```python
from build123d import *

# Parameters (mm, degrees)
F0_W     = 111
F0_H     = 7
F2_W     = 4.5
F2_H     = 2.05
F3_DEPTH = 12.5
F4_SIZE  = 0.5


with BuildPart() as f1:
    # F0 (on Front) → F1 (revolve)
    with BuildSketch(Plane.XZ):
        with Locations((55.5, 3.5)):
            Rectangle(F0_W, F0_H)
    revolve(axis=Axis((55.5, 0, 0), (-1, 0, 0)))

    # F2 (on Front) → F3 (cut, symmetric)
    with BuildSketch(Plane.XZ):
        with Locations((2.25, 5.975)):
            Rectangle(F2_W, F2_H)
        with Locations((2.25, -5.975)):
            Rectangle(F2_W, F2_H)
    extrude(amount=F3_DEPTH, both=True, mode=Mode.SUBTRACT)

    # F4
    f4_edges = [f1.edges().sort_by_distance(p)[0] for p in [
        (0, -7, 0),
        (0, 7, 0),
        (111, 0, -7),
    ]]
    chamfer(f4_edges, length=F4_SIZE)


solid = f1.part
```
The model under review builds one solid part; all positions refer to its coordinate system, in mm. A direction names the side the tool comes from. Give positions to 0.01 mm unless a question says otherwise; leave off trailing zeros. Write each loop counter-clockwise with the first axis right and the second up, starting at its lowest first coordinate (ties: lowest second). Pieces come first, ordered by that corner, then holes. Notation, with made-up numbers: M 73.25,-14 L 78.25,-14 A6 ccw 78.25,-10 Z; hole C -9,-11.5 d11. An arc over 180 degrees is marked long. Write item = value, one per line. Start each with the question number.
Q1. Machinability: for faces 1 (the face through (4.5, 0, -6)), 2 (the face through (0.14, 6.64, 0.08)), 3 (the face through (2, 0, 4.95)), which of the approach directions +Z, -Z, +X, -X, +Y, -Y give a long, thin tool a straight path to every point of the face, cutting with its end or side? Answer none if there is none.
Q2. For line 1 (Y direction, x = 29.5, z = 0.5); line 2 (X direction, y = -3.25, z = 5.5); line 3 (Z direction, x = 7, y = 0.25), list the stretches that pass through material, from the lowest coordinate up.
Q3. We need section A-A (x = 49.5). State the section outline as (y, z) points, plus the area to 3 significant figures.
Q4. Clearance check with flat-ended pins moving along their axes: pin 1 (3 mm diameter, centred on x = 32, z = -4, fed in from +Y); pin 2 (3.5 mm diameter, centred on x = 2, y = -0.5, fed in from +Z); pin 3 (1 mm diameter, centred on y = 0, z = -6, fed in from -X). State where each tip first meets the part, or that it passes through.
Result set:
q1.face_1 = -Z, -X, +Y, -Y
q1.face_2 = -X, +Y
q1.face_3 = +Z, -X, +Y, -Y
q2.line_1 = -6.98 to 6.98
q2.line_2 = 4.5 to 111
q2.line_3 = -7 to 7
q3.outline = C 0,0 d14
q3.area = 154 mm2
q4.pin_1 = 6.54
q4.pin_2 = 4.95
q4.pin_3 = 4.5
